Work out the finished part from the listing and answer in its coordinate system (mm). A direction names the side the tool comes from. Coordinates: 2 decimals unless noted, no trailing zeros. Loops run counter-clockwise (first coordinate to the right, second up) from the corner with the lowest first, then second, coordinate; pieces in that order, holes last. Notation, with made-up numbers: (79.5, 51) -> (138.5, 51) arc R28 ccw to (138.5, 87) -> close; hole circle Ø2 at (14.5, -34). An arc over 180 degrees is marked (long way). Answer as CSV lines item,"result".
```python
from build123d import *

# Parameters (mm, degrees)
SKETCH1_R               = 40
BOSS_EXTRUDE1_DEPTH     = 24
SKETCH2_W               = 80
SKETCH2_H               = 80
SKETCH2_R               = 2
BOSS_EXTRUDE2_DEPTH     = 5
FILLET1_R               = 4
SKETCH3_R               = 34
BOSS_EXTRUDE3_DEPTH     = 100
FILLET2_R               = 4
SKETCH4_R               = 10
BOSS_EXTRUDE4_DEPTH     = 3
SKETCH5_R               = 5
BOSS_EXTRUDE5_DEPTH     = 50
FILLET3_R               = 1
FILLET4_R               = 1
SKETCH6_W               = 26.979088542
SKETCH6_H               = 2
CUT_EXTRUDE1_DEPTH      = 1
CUT_EXTRUDE1_DEPTH_BACK = 81
SKETCH8_R               = 2
BOSS_EXTRUDE6_DEPTH     = 7
FILLET5_R               = 2


with BuildPart() as part:
    # Sketch1 → Boss-Extrude1 (new body)
    with BuildSketch(Plane.XY):
        Circle(SKETCH1_R)
    extrude(amount=BOSS_EXTRUDE1_DEPTH)

    # Sketch2 → Boss-Extrude2 (add)
    with BuildSketch(Plane.XY.offset(24)):
        Rectangle(SKETCH2_W, SKETCH2_H)
        with Locations((33, -33)):
            Circle(SKETCH2_R, mode=Mode.SUBTRACT)
        with Locations((-33, 33)):
            Circle(SKETCH2_R, mode=Mode.SUBTRACT)
        with Locations((33, 33)):
            Circle(SKETCH2_R, mode=Mode.SUBTRACT)
        with Locations((-33, -33)):
            Circle(SKETCH2_R, mode=Mode.SUBTRACT)
    extrude(amount=BOSS_EXTRUDE2_DEPTH)

    # Fillet1
    fillet1_edges = [part.edges().sort_by_distance(p)[0] for p in [
        (40, 40, 26.5),
        (-40, 40, 26.5),
        (-40, -40, 26.5),
        (40, -40, 26.5),
    ]]
    fillet(fillet1_edges, radius=FILLET1_R)

    # Sketch3 → Boss-Extrude3 (add)
    with BuildSketch(Plane(origin=(0, 0, 0), x_dir=(-1, 0, 0), z_dir=(0, 0, -1))):
        Circle(SKETCH3_R)
    extrude(amount=BOSS_EXTRUDE3_DEPTH)

    # Fillet2
    fillet2_edges = [part.edges().sort_by_distance(p)[0] for p in [
        (-40, 0, 0),
        (34, 0, -100),
    ]]
    fillet(fillet2_edges, radius=FILLET2_R)

    # Sketch4 → Boss-Extrude4 (add)
    with BuildSketch(Plane.XY.offset(29)):
        with Locations((0, -15)):
            Circle(SKETCH4_R)
    extrude(amount=BOSS_EXTRUDE4_DEPTH)

    # Sketch5 → Boss-Extrude5 (add)
    with BuildSketch(Plane.XY.offset(32)):
        with Locations((0, -15)):
            Circle(SKETCH5_R)
    extrude(amount=BOSS_EXTRUDE5_DEPTH)

    # Fillet3
    fillet3_edges = [part.edges().sort_by_distance(p)[0] for p in [
        (-10, -15, 32),
    ]]
    fillet(fillet3_edges, radius=FILLET3_R)

    # Fillet4
    fillet4_edges = [part.edges().sort_by_distance(p)[0] for p in [
        (-5, -15, 82),
    ]]
    fillet(fillet4_edges, radius=FILLET4_R)

    # Sketch6 → Cut-Extrude1 (cut, two sides)
    with BuildSketch(Plane.ZY.offset(40)) as cut_extrude1_sk:
        with Locations((75.489544271, -11)):
            Rectangle(SKETCH6_W, SKETCH6_H)
    extrude(amount=CUT_EXTRUDE1_DEPTH, mode=Mode.SUBTRACT)
    extrude(cut_extrude1_sk.sketch, amount=-CUT_EXTRUDE1_DEPTH_BACK, mode=Mode.SUBTRACT)

    # Sketch8 → Boss-Extrude6 (add)
    with BuildSketch(Plane.XY.offset(29)):
        with BuildLine():
            Line((-36, -24), (-40, -24))
            Line((-40, -24), (-40, -36))
            ThreePointArc((-40, -36), (-38.828427125, -38.828427125), (-36, -40))
            Line((-36, -40), (-29, -40))
            Line((-29, -40), (-29, -32))
            Line((-29, -32), (-36, -24))
        make_face()
        with Locations((-33, -33)):
            Circle(SKETCH8_R, mode=Mode.SUBTRACT)
        with BuildLine():
            Line((29, -32), (29, -40))
            Line((29, -40), (36, -40))
            ThreePointArc((36, -40), (38.828427125, -38.828427125), (40, -36))
            Line((40, -36), (40, -24))
            Line((40, -24), (36, -24))
            Line((36, -24), (29, -32))
        make_face()
        with Locations((33, -33)):
            Circle(SKETCH8_R, mode=Mode.SUBTRACT)
        with BuildLine():
            Line((-40, 36), (-40, 24))
            Line((-40, 24), (-36, 24))
            Line((-36, 24), (-29, 32))
            Line((-29, 32), (-29, 40))
            Line((-29, 40), (-36, 40))
            ThreePointArc((-36, 40), (-38.828427125, 38.828427125), (-40, 36))
        make_face()
        with Locations((-33, 33)):
            Circle(SKETCH8_R, mode=Mode.SUBTRACT)
        with BuildLine():
            Line((36, 40), (29, 40))
            Line((29, 40), (29, 32))
            Line((29, 32), (36, 24))
            Line((36, 24), (40, 24))
            Line((40, 24), (40, 36))
            ThreePointArc((40, 36), (38.828427125, 38.828427125), (36, 40))
        make_face()
        with Locations((33, 33)):
            Circle(SKETCH8_R, mode=Mode.SUBTRACT)
    extrude(amount=BOSS_EXTRUDE6_DEPTH)

    # Fillet5
    fillet5_edges = [part.edges().sort_by_distance(p)[0] for p in [
        (-36, -24, 32.5),
        (-40, -24, 32.5),
        (-29, -40, 32.5),
        (-29, -32, 32.5),
        (36, -24, 32.5),
        (29, -32, 32.5),
        (29, -40, 32.5),
        (40, -24, 32.5),
        (-36, 24, 32.5),
        (-29, 32, 32.5),
        (-29, 40, 32.5),
        (-40, 24, 32.5),
        (36, 24, 32.5),
        (40, 24, 32.5),
        (29, 40, 32.5),
        (29, 32, 32.5),
    ]]
    fillet(fillet5_edges, radius=FILLET5_R)


solid = part.part
```
(1) For a pull along X with two mould halves and no side action, classify faces 1 (the face through (33.923, 31.226, 29.916)), 2 (the face through (-18.28, 28.67, -47.33)), 3 (the face through (-1, 40, 27)) as pulls with the +X half, pulls with the -X half, needs draft (parallel to the pull), parting line crosses it, or undercut.
Computed values:
face 1,"undercut"
face 2,"parting line crosses it"
face 3,"needs draft"
(2) A cutting plane is placed at A-A, the plane z = 58. Write down the section's boundary in (x, y).
Computed values:
outline,"circle Ø10 at (0, -15)"
(3) A cutting plane is placed at B-B, the plane z = -19. Write down the section's boundary in (x, y), and give its area (3 significant figures).
Computed values:
outline,"circle Ø68 at (0, 0)"
area,"3,630 mm2"
(4) Consider line 1 along Y through (x, z) = (33, 28); line 2 along Y through (x, z) = (33, 33.5); line 3 along Z through (x, y) = (-23, -19.5). Determine where each line is inside the solid, lowest interval first.
Computed values:
line 1,"-40 to -35, -31 to 31, 35 to 40"
line 2,"-40 to -35, -31 to -27.43, 27.43 to 31, 35 to 40"
line 3,"-100 to 29"
(5) Flat-ended cylindrical pins translate along their axes: pin 1 Ø5.5 at (x, y) = (36.5, -35) entering from +Z; pin 2 Ø1.5 at (y, z) = (24, 2) entering from +X; pin 3 Ø4 at (x, z) = (-1, 68.5) entering from +Y. Find the tip coordinate at first contact, or state that the pin passes through.
Computed values:
pin 1,"z = 36"
pin 2,"x = 32.06"
pin 3,"y = -12"
(6) Which of the six approach directions +Z, -Z, +X, -X, +Y, -Y give full straight-line access (tool end or side, diameter ignored) to faces 4 (the face through (30, -30, 24)), 5 (the face through (-29, -35, 32)), 6 (the face through (-1.302, -5.085, 29.986)), 7 (the face through (32, -13, 0)), 8 (the face through (30, 30, 24))?
Computed values:
face 4,"-Z, +X, -Y"
face 5,"+Z, +Y, -Y"
face 6,"+Z"
face 7,"-Z"
face 8,"-Z, +X, +Y"
